Verification items for the finished model (mm, model axes). A direction names the side the tool comes from. Coordinates: 2 decimals unless noted, no trailing zeros. Loops run counter-clockwise (first coordinate to the right, second up) from the corner with the lowest first, then second, coordinate; pieces in that order, holes last. Notation, with made-up numbers: (14.25, 65.25) -> (36.25, 65.25) arc R27 cw to (36.25, 103.25) -> close; hole circle Ø1 at (-38.5, -33.5). An arc over 180 degrees is marked (long way). Write item = value, one per line.
```python
from build123d import *

# Parameters (mm, degrees)
SKETCH2_W                    = 95.25
SKETCH2_H                    = 63.5
BASE_FLANGE1_DEPTH           = 4.7752
EDGE_FLANGE1_STRIP_CUT_DEPTH = 63.5
EDGE_FLANGE1_DEPTH           = 63.5
FILLET1_R                    = 6.35
SKETCH10_W                   = 26.9875
SKETCH10_H                   = 7.9375
CUT_EXTRUDE1_DEPTH           = 117.826050987
FILLET2_R                    = 0.396875


# Sheet-metal steps are written as plain solids
with BuildPart() as part:
    # Sketch2 → Base-Flange1 (new body)
    with BuildSketch(Plane(origin=(0, 0, 0), x_dir=(1, 0, 0), z_dir=(0, 1, 0))):
        with Locations((47.625, 31.75)):
            Rectangle(SKETCH2_W, SKETCH2_H)
    extrude(amount=-BASE_FLANGE1_DEPTH)

    # Edge-Flange1 strip (across the edge) → Edge-Flange1 strip cut (cut)
    with BuildSketch(Plane(origin=(0, 0, -63.5), x_dir=(0.3090169943749416, 0.9510565162951554, 0), z_dir=(0, 0, 1))):
        Polygon((-13.826403209, 27.100421727), (-4.250584587, -2.3709176), (0.29090049, -0.895299648), (-9.284918132, 28.576039679), align=None)
    extrude(amount=EDGE_FLANGE1_STRIP_CUT_DEPTH, mode=Mode.SUBTRACT)

    # Edge-Flange1 section (across the edge) → Edge-Flange1 (add)
    with BuildSketch(Plane(origin=(0, 0, -63.5), x_dir=(0.3090169943749416, 0.9510565162951554, 0), z_dir=(0, 0, 1))):
        with BuildLine():
            Line((-4.7752, 0.94137376), (-4.7752, 75.443682621))
            Line((-4.7752, 75.443682621), (0, 75.443682621))
            Line((0, 75.443682621), (0, 0.94137376))
            ThreePointArc((0, 0.94137376), (0.073175579, 0.011589873), (0.29090049, -0.895299648))
            Line((0.29090049, -0.895299648), (-4.250584587, -2.3709176))
            ThreePointArc((-4.250584587, -2.3709176), (-4.643233785, -0.735415984), (-4.7752, 0.94137376))
        make_face()
    extrude(amount=EDGE_FLANGE1_DEPTH)

    # Fillet1
    fillet1_edges = [part.edges().sort_by_distance(p)[0] for p in [
        (-72.489014945, 21.04263751, -63.5),
        (-72.489014945, 21.04263751, 0),
        (95.25, -2.3876, -63.5),
        (95.25, -2.3876, 0),
    ]]
    fillet(fillet1_edges, radius=FILLET1_R)

    # Sketch10 → Cut-Extrude1 (cut, through all)
    with BuildSketch(Plane(origin=(0, 0, 0), x_dir=(1, 0, 0), z_dir=(0, 1, 0))):
        with Locations((27.13512376, 31.75)):
            Rectangle(SKETCH10_W, SKETCH10_H)
    extrude(amount=-CUT_EXTRUDE1_DEPTH, mode=Mode.SUBTRACT)

    # Fillet2
    fillet2_edges = [part.edges().sort_by_distance(p)[0] for p in [
        (13.64137376, -2.3876, -27.78125),
        (13.64137376, -2.3876, -35.71875),
        (40.62887376, -2.3876, -35.71875),
        (40.62887376, -2.3876, -27.78125),
    ]]
    fillet(fillet2_edges, radius=FILLET2_R)


solid = part.part
```
1) Sectioned sample at A-A, the plane x = 23. Record the cut outline in (y, z), plus the area to 3 significant figures.
Ans:
outline = (-4.78, -63.5) -> (0, -63.5) -> (0, -35.72) -> (-4.78, -35.72) -> close; (-4.78, -27.78) -> (0, -27.78) -> (0, 0) -> (-4.78, 0) -> close
area = 265 mm2
2) Sectioned sample at B-B, the plane z = -48.5. Record the cut outline in (x, y), plus the area to 3 significant figures.
Ans:
outline = (-73.23, 18.77) -> (-2.37, -4.25) arc R10.72 ccw to (0.94, -4.78) -> (95.25, -4.78) -> (95.25, 0) -> (0.94, 0) arc R5.94 cw to (-0.9, 0.29) -> (-71.75, 23.31) -> close
area = 819 mm2
3) Depth check by flat-ended pin: pin 1 Ø4 at (x, z) = (-9, -40) entering from +Y; pin 2 Ø2 at (x, z) = (-32.5, -8) entering from -Y; pin 3 Ø19 at (x, z) = (67, -47) entering from +Y. Enter the tip coordinate at first touch or a pass-through.
Ans:
pin_1 = 3.57
pin_2 = 5.21
pin_3 = 0
4) Material ranges on line 1 (Y direction, x = 36.5, z = -45); line 2 (Y direction, x = -20, z = -17.5), recorded low to high.
Ans:
line_1 = -4.78 to 0
line_2 = 1.48 to 6.5
5) Tool access check on faces 4 (the face through (47, -4.775, -32)), 5 (the face through (13.641, -2, -32)). Record the directions out of +Z, -Z, +X, -X, +Y, -Y that give a thin tool (end or side, any length) a straight path to the whole face; none if there is none.
Ans:
face_4 = +Z, -Z, +X, -X, -Y
face_5 = +Y, -Y
6) Sectioned sample at D-D, the plane y = 9.25. Record the cut outline in (x, z), plus the area to 3 significant figures.
Ans:
outline = (-43.92, -63.5) -> (-28.47, -63.5) -> (-28.47, 0) -> (-43.92, 0) -> close
area = 981 mm2
7) Sectioned sample at C-C, the plane x = 6. Record the cut outline in (y, z).
Ans:
outline = (-4.78, -63.5) -> (0, -63.5) -> (0, 0) -> (-4.78, 0) -> close
8) Release check for a two-part mould opening along Z. For faces 1 (the face through (47, 0, -32)), 2 (the face through (8, -1, 0)), 3 (the face through (40.629, -2, -32)) record: pulls with the +Z half, pulls with the -Z half, needs draft (parallel to the pull), parting line crosses it, or undercut.
Ans:
face_1 = needs draft
face_2 = pulls with the +Z half
face_3 = undercut
